from build123d import *

# Parameters (mm, degrees)
BOSS_EXTRUDE1_DEPTH = 20
SKETCH3_R           = 3
CUT_EXTRUDE1_DEPTH  = 4
BOSS_EXTRUDE2_DEPTH = 12
SKETCH5_R           = 1
CUT_EXTRUDE2_DEPTH  = 17
BOSS_EXTRUDE3_DEPTH = 17
SKETCH10_R          = 6.25
CUT_EXTRUDE3_DEPTH  = 4
BOSS_EXTRUDE4_DEPTH = 10


with BuildPart() as part:
    # Sketch2 → Boss-Extrude1 (new body)
    with BuildSketch(Plane(origin=(0, 0, 0), x_dir=(1, 0, 0), z_dir=(0, 1, 0))):
        Polygon((-29.519694138, 7.160148579), (-29.519694138, -17.339851421), (-23.519694138, -17.339851421), (-23.519694138, -14.339851421), (-25.519694138, -14.339851421), (-25.519694138, 4.160148579), (-23.519694138, 4.160148579), (-23.519694138, 7.160148579), align=None)
    extrude(amount=BOSS_EXTRUDE1_DEPTH)

    # Sketch3 → Cut-Extrude1 (cut)
    with BuildSketch(Plane.ZY.offset(29.519694138)):
        with Locations((5.089851421, 11)):
            Circle(SKETCH3_R)
    extrude(amount=-CUT_EXTRUDE1_DEPTH, mode=Mode.SUBTRACT)

    # Sketch4 → Boss-Extrude2 (add)
    with BuildSketch(Plane.XZ):
        Polygon((-16.519694138, -3.410148579), (-33.519694138, -3.410148579), (-33.519694138, 13.589851421), (-16.519694138, 13.589851421), (-16.519694138, 10.089851421), (-30.019694138, 10.089851421), (-30.019694138, 0.089851421), (-16.519694138, 0.089851421), align=None)
    extrude(amount=BOSS_EXTRUDE2_DEPTH)

    # Sketch5 → Cut-Extrude2 (cut)
    with BuildSketch(Plane(origin=(0, 0, -3.410148579), x_dir=(-1, 0, 0), z_dir=(0, 0, -1))):
        with Locations((19.019694138, -7.8)):
            Circle(SKETCH5_R)
        with Locations((27.019694138, -7.8)):
            Circle(SKETCH5_R)
    extrude(amount=-CUT_EXTRUDE2_DEPTH, mode=Mode.SUBTRACT)

    # Sketch6 → Boss-Extrude3 (add)
    with BuildSketch(Plane(origin=(0, 0, -3.410148579), x_dir=(-1, 0, 0), z_dir=(0, 0, -1))):
        Polygon((33.519694138, 0), (29.519694138, 19.957202976), (29.519694138, 0), align=None)
    extrude(amount=-BOSS_EXTRUDE3_DEPTH)

    # Sketch10 → Cut-Extrude3 (cut)
    with BuildSketch(Plane.ZY.offset(29.519694138)):
        with Locations(Location((5.089851421, 11, 0), (0, 0, 90))):
            Circle(SKETCH10_R)
    extrude(amount=CUT_EXTRUDE3_DEPTH, mode=Mode.SUBTRACT)

    # Sketch11 → Boss-Extrude4 (add)
    with BuildSketch(Plane(origin=(0, 0, 10.089851421), x_dir=(-1, 0, 0), z_dir=(0, 0, -1))):
        Polygon((25.519694138, 0), (30.019694138, -3.647368963), (30.019694138, 0), align=None)
    extrude(amount=BOSS_EXTRUDE4_DEPTH)


solid = part.part
Check sheet for the modelled part. Datum: model origin and axes. Units: mm. A direction names the side the tool comes from. Give positions to 0.01 mm unless a question says otherwise; leave off trailing zeros. Write each loop counter-clockwise with the first axis right and the second up, starting at its lowest first coordinate (ties: lowest second). Pieces come first, ordered by that corner, then holes. Notation, with made-up numbers: M 42,23 L 83,23 A9 cw 83,33 Z; hole C 47.5,1 d1. An arc over 180 degrees is marked long. Use one line per item in the form item = value.
(1) Section check D-D on y = -4.5. Record the boundary of the cut face in (x, z), plus the area to 3 significant figures.
Answer block:
outline = M -33.52,-3.41 L -16.52,-3.41 L -16.52,0.09 L -30.02,0.09 L -30.02,10.09 L -16.52,10.09 L -16.52,13.59 L -33.52,13.59 Z
area = 154 mm2
(2) Depth check by flat-ended pin: P1, Ø2, axis at x = -19, y = 0, coming from the -Z side; P2, Ø6, axis at x = -21.5, y = -8, coming from the +Z side; P3, Ø1.2, axis at x = -27.02, y = -7.8, coming from the -Z side; P4, Ø5, axis at x = -19, z = 9, coming from the +Y side. Enter the tip coordinate at first touch or a pass-through.
Answer block:
P1 = -3.41
P2 = 13.59
P3 = through
P4 = 0
(3) Section check B-B on x = -24.25. Record the boundary of the cut face in (y, z).
Answer block:
outline = M -12,-3.41 L 0,-3.41 L 0,0.09 L -12,0.09 Z; M -12,10.09 L 0,10.09 L 0,13.59 L -12,13.59 Z; M 0,-7.16 L 20,-7.16 L 20,-4.16 L 0,-4.16 Z; M 0,14.34 L 20,14.34 L 20,17.34 L 0,17.34 Z
(4) Tool access check on faces 4 (the flat face through (-25, 10, -4.16)), 5 (the flat face through (-25.52, 7.6, 5.2)), 6 (the flat face through (-27, 0, -5)). Record the directions out of +Z, -Z, +X, -X, +Y, -Y that give a thin tool (end or side, any length) a straight path to the whole face; none if there is none.
Answer block:
face_4 = +X, +Y, -Y
face_5 = +X, +Y
face_6 = -Z, +X, -X, -Y
(5) Draft check along X on faces 1 (the cylindrical face through (-26.02, -7.76, -1.68)), 2 (the flat face through (-25, 10, 14.34)), 3 (the flat face through (-30.02, -8, 5)). Enter one of: pulls with the +X half, pulls with the -X half, needs draft (parallel to the pull), parting line crosses it, or undercut.
Answer block:
face_1 = undercut
face_2 = needs draft
face_3 = pulls with the +X half
(6) Section check C-C on z = 3.25. Record the boundary of the cut face in (x, y).
Answer block:
outline = M -33.52,-12 L -30.02,-12 L -30.02,-3.65 L -25.52,0 L -25.52,8.63 L -29.52,8.63 L -29.52,5.03 L -32.51,5.03 L -33.52,0 Z; M -30.12,16.97 L -29.52,16.97 L -29.52,13.37 L -25.52,13.37 L -25.52,20 L -29.52,20 L -29.52,19.96 Z
(7) Section check A-A on y = -7.8. Record the boundary of the cut face in (x, z).
Answer block:
outline = M -33.52,-3.41 L -28.02,-3.41 L -28.02,0.09 L -30.02,0.09 L -30.02,10.09 L -28.02,10.09 L -28.02,13.59 L -33.52,13.59 Z; M -26.02,-3.41 L -20.02,-3.41 L -20.02,0.09 L -26.02,0.09 Z; M -26.02,10.09 L -20.02,10.09 L -20.02,13.59 L -26.02,13.59 Z; M -18.02,-3.41 L -16.52,-3.41 L -16.52,0.09 L -18.02,0.09 Z; M -18.02,10.09 L -16.52,10.09 L -16.52,13.59 L -18.02,13.59 Z
(8) Material ranges on line 1 along Z through (x, y) = (-18.5, -1); line 2 along X through (y, z) = (7.5, 9); line 3 along Z through (x, y) = (-30.75, 4), recorded low to high.
Answer block:
line_1 = -3.41 to 0.09, 10.09 to 13.59
line_2 = -29.52 to -25.52
line_3 = -3.41 to 13.59
